Autodesk Inventor part; units mm, degrees
ref_plane "YZ Plane" through (0, 0, 0) normal (1, 0, 0) x (0, 1, 0)
ref_plane "XZ Plane" through (0, 0, 0) normal (0, 1, 0) x (-1, 0, 0)
ref_plane "XY Plane" through (0, 0, 0) normal (0, 0, 1) x (1, 0, 0)
sketch "Sketch1" plane through (0, 0, 0) normal (0, 0, 1) x (1, 0, 0)
  circle A0 centre (0, 0) radius 20.955
  circle A1 centre (0, 0) radius 18.415
  arc A2 (1.196, 17.1032) -> (-1.196, 17.1032) centre (0, 0) ccw
  line L0 (0, 0) -> (0, 27.5348)
  line L1 (1.196, 17.1032) -> (1.2846, 18.3701)
  line L2 (-1.196, 17.1032) -> (-1.2846, 18.3701)
  dimension "d0" = 41.91
  dimension "d2" = 1.27
  dimension "d3" = 2.54
extrude "Extrusion1" add sketch "Sketch1" along normal blind 12.7
extrude "Extrusion2" add sketch "Sketch1" along normal blind 12.7 contours A1 L1 A2 L0 | L0 A2 L2 A1
pattern_circular "Circular Pattern1" count 15 over 360 about axis through (0, 0, 0) along (0, 0, 1) of "Extrusion2", "Extrusion1"
properties part number "AWAutomobloxTire"
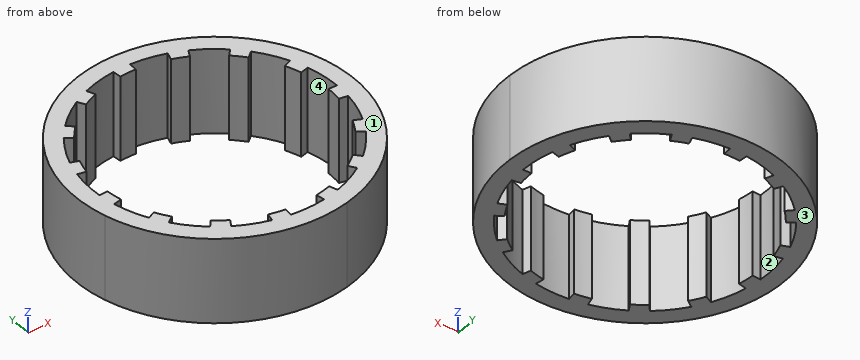
Read the model definition and answer for the solid it produces. Units are mm, in the model's axes. Face numbers are marked on the shaded views. A direction names the side the tool comes from. Coordinates: 2 decimals unless noted, no trailing zeros. Write each loop counter-clockwise with the first axis right and the second up, starting at its lowest first coordinate (ties: lowest second). Pieces come first, ordered by that corner, then holes. Notation, with made-up numbers: (29, 8.25) -> (49, 8.25) arc R25 cw to (49, 26.25) -> close; hole circle Ø4 at (41, 83.25). An arc over 180 degrees is marked (long way). Answer as a JSON object with one key per item and string values.
Q1. The part is cut by section B-B on x = -7. Give the vertices of the cut face in (y, z).
The answers:
{"outline": "(-19.75, 0) -> (-17.03, 0) -> (-17.03, 12.7) -> (-19.75, 12.7) -> close; (15.65, 0) -> (19.75, 0) -> (19.75, 12.7) -> (15.65, 12.7) -> close"}
Q2. Determine the mould class of the marked faces 1 and 2 for opening direction X: pulls with the +X half, pulls with the -X half, needs draft (parallel to the pull), parting line crosses it, or undercut.
The answers:
{"face 1": "needs draft", "face 2": "undercut"}
Q3. Consider line 1 (X direction, y = 12, z = 2.25); line 2 (Y direction, x = -4, z = 8.75); line 3 (Y direction, x = -12, z = 1.5). Determine where each line is inside the solid, lowest interval first. Write a range as [from, to].
The answers:
{"line 1": "x = [-17.18, -12.25], [12.25, 17.18]", "line 2": "y = [-20.57, -16.67], [17.98, 20.57]", "line 3": "y = [-17.18, -13.97], [12.25, 12.43], [13.97, 17.18]"}
Q4. A tool of negligible diameter and unlimited length cuts with its end or side. For the marked faces 3 and 4, from which of +Z, -Z, +X, -X, +Y, -Y can it reach the whole face along a straight path? Write none if from no direction.
The answers:
{"face 3": "-Z, +X, -X, +Y, -Y", "face 4": "+Z, -Z"}
Q5. The part is cut by section A-A on x = 0. Give the vertices of the cut face in (y, z) (3 decimals).
The answers:
{"outline": "(-20.955, 0) -> (-18.415, 0) -> (-18.415, 12.7) -> (-20.955, 12.7) -> close; (17.145, 0) -> (20.955, 0) -> (20.955, 12.7) -> (17.145, 12.7) -> close"}
Q6. Flat-ended cylindrical pins translate along their axes: pin 1 Ø6 at (y, z) = (-16.5, 7.5) entering from -X; pin 2 Ø4 at (x, z) = (-1, 4) entering from +Y (3 decimals); pin 3 Ø6 at (y, z) = (-10.5, 6.5) entering from +X. Find the tip coordinate at first contact, or state that the pin passes through.
The answers:
{"pin 1": "stops at x = -16.03", "pin 2": "stops at y = 20.955", "pin 3": "stops at x = 19.57"}
